```python
from build123d import *

# Parameters (mm, degrees)
BOSS_EXTRUDE1_DEPTH     = 38.1
F_1_4_CLEARANCE_HOLE1_D = 6.7564


with BuildPart() as part:
    # Sketch1 → Boss-Extrude1 (new body, symmetric)
    with BuildSketch(Plane.XY):
        Polygon((28.575, -47.625), (31.75, -47.625), (31.75, 3.175), (-31.75, 3.175), (-31.75, -47.625), (-28.575, -47.625), (-28.575, 0), (28.575, 0), align=None)
    extrude(amount=BOSS_EXTRUDE1_DEPTH, both=True)

    # 1/4 Clearance Hole1 (through all)
    with Locations(Plane(origin=(0, 3.175, 0), x_dir=(1, 0, 0), z_dir=(0, 1, 0))):
        with Locations((-19.05, 25.4), (19.05, 25.4), (19.05, -25.4), (-19.05, -25.4)):
            Hole(F_1_4_CLEARANCE_HOLE1_D / 2)


solid = part.part
```
Input: part model. Units: mm. Frame: model coordinates. A direction names the side the tool comes from. Round coordinates to 2 decimals unless told otherwise and drop trailing zeros. Order: outer loops, then holes, each group sorted by start corner. A loop starts at its lowest first (then second) coordinate and runs counter-clockwise, first axis right, second up. Notation, with made-up numbers: (-11.75, 44) - (8.25, 44) arc R25 ccw to (8.25, 67) - close; hole circle Ø4 at (80.5, -6). An arc over 180 degrees is marked (long way). One line per question, with ' | ' between items. Start each with the question number.
1) Cut plane C-C, the plane z = -25.4. Return the cut outline in (x, y) (3 decimals), then the cut area to 3 significant figures.
2) Set-up query: faces 1 (the flat face through (28.575, -23, 1)), 2 (the cylindrical face through (-18.32, 1.57, 28.7)). Return all of +Z, -Z, +X, -X, +Y, -Y with unobstructed straight access to the full face (end or side cutting, diameter ignored); none if empty.
3) Cut plane D-D, the plane x = 7. Return the cut outline in (y, z) (3 decimals).
4) Contact query for a flat-ended pin moving along its axis: P1, Ø17, axis at x = -1, z = 17.5, coming from the -Y side. Output: stop coordinate, or through.
5) Ray query, probe 1 along X at (y, z) = (0.75, 25.4); probe 2 along Z at (x, y) = (19, 2); probe 3 along X at (y, z) = (-12, -31.5) (3 decimals). Return the intervals inside material, ascending.
6) Cut plane A-A, the plane y = -26. Return the cut outline in (x, z) (3 decimals).
7) Pull-direction query (X, two-part tool) for faces 3 (the flat face through (0, 0, 1)), 4 (the cylindrical face through (19.78, 1.57, -22.1)), 5 (the flat face through (0, 3.175, 1)), 6 (the flat face through (-31.75, -22, 1)); classes: +X half, -X half, draft (parallel to the pull), parting line (faces both ways), or undercut.
8) Cut plane B-B, the plane x = -19.05. Return the cut outline in (y, z) (3 decimals).
Worked out:
1) outline: (-31.75, -47.625) - (-28.575, -47.625) - (-28.575, 0) - (-22.428, 0) - (-22.428, 3.175) - (-31.75, 3.175) - close; (-15.672, 0) - (15.672, 0) - (15.672, 3.175) - (-15.672, 3.175) - close; (22.428, 0) - (28.575, 0) - (28.575, -47.625) - (31.75, -47.625) - (31.75, 3.175) - (22.428, 3.175) - close | area: 461 mm^2
2) face 1: +Z, -Z, -Y | face 2: +Y, -Y
3) outline: (0, -38.1) - (3.175, -38.1) - (3.175, 38.1) - (0, 38.1) - close
4) P1: stops at y = 0
5) probe 1: x = -31.75 to -22.43, -15.67 to 15.67, 22.43 to 31.75 | probe 2: z = -38.1 to -28.78, -22.02 to 22.02, 28.78 to 38.1 | probe 3: x = -31.75 to -28.575, 28.575 to 31.75
6) outline: (-31.75, -38.1) - (-28.575, -38.1) - (-28.575, 38.1) - (-31.75, 38.1) - close; (28.575, -38.1) - (31.75, -38.1) - (31.75, 38.1) - (28.575, 38.1) - close
7) face 3: undercut | face 4: undercut | face 5: draft | face 6: -X half
8) outline: (0, -38.1) - (3.175, -38.1) - (3.175, -28.778) - (0, -28.778) - close; (0, -22.022) - (3.175, -22.022) - (3.175, 22.022) - (0, 22.022) - close; (0, 28.778) - (3.175, 28.778) - (3.175, 38.1) - (0, 38.1) - close
